Here's how the part is built. I have some questions about the finished solid (model axes, mm). Give positions to 0.01 mm unless a question says otherwise; leave off trailing zeros. Loops run counter-clockwise (first coordinate to the right, second up) from the corner with the lowest first, then second, coordinate; pieces in that order, holes last.
Q1. Suppose I cut it at C-C (x = 75.5). List the corners of the cut face in (y, z) for me (3 decimals).
Q2. I'm going to push flat-ended pins straight in: P1, Ø2, axis at x = 95, y = 1.5, coming from the -Z side; P2, Ø2.5, axis at x = 10.32, z = 0, coming from the +Y side; P3, Ø3, axis at x = -12, y = 0, coming from the +Z side; P4, Ø1, axis at y = 2, z = 62.5, coming from the +X side. Where does each tip first touch, or does it pass through?
Q3. Suppose I cut it at A-A (y = 1.25). Count the separate pieces of the cut face and the enclosed holes in it, and give its area (3 significant figures).
Q4. Thinking about a two-plate mould opening in Y: for faces 1 (the face through (2, -3.175, -2)), 2 (the face through (2, 3.175, -2)), 3 (the face through (-92.73, 0.04, -120.94)), which applies, pulls with the +Y half, pulls with the -Y half, needs draft (parallel to the pull), parting line crosses it, or undercut?
Q5. I need wall thicknesses on probe 1 along X at (y, z) = (-0.25, 0); probe 2 along Z at (x, y) = (87, -1.5); probe 3 along Z at (x, y) = (101.6, 1). Which ranges of each line are inside material? Lowest first, please.
Q6. Suppose I cut it at B-B (z = 65.5). List the corners of the cut face in (x, y) for me (3 decimals).
```python
from build123d import *

# Parameters (mm, degrees)
SKETCH1_R           = 152.4
BOSS_EXTRUDE1_DEPTH = 3.175
SKETCH3_R           = 2.20345
CUT_EXTRUDE1_DEPTH  = 216.619670949
SKETCH5_R           = 1.524
CUT_EXTRUDE3_DEPTH  = 216.619670949


with BuildPart() as part:
    # Sketch1 → Boss-Extrude1 (new, symmetric)
    with BuildSketch(Plane(origin=(0, 0, 0), x_dir=(1, 0, 0), z_dir=(0, 1, 0))):
        with Locations(Location((0, 0, 0), (0, 0, 270))):
            Circle(SKETCH1_R)
    extrude(amount=BOSS_EXTRUDE1_DEPTH, both=True)

    # Sketch3 → Cut-Extrude1 (cut, through all)
    with BuildSketch(Plane(origin=(0, 3.175, 0), x_dir=(1, 0, 0), z_dir=(0, 1, 0))):
        with Locations(Location((-10.31875, 0, 0), (0, 0, 270))):
            Circle(SKETCH3_R)
        with Locations(Location((10.31875, 0, 0), (0, 0, 270))):
            Circle(SKETCH3_R)
        with Locations(Location((66.013427029, 76.332177029, 0), (0, 0, 270))):
            Circle(SKETCH3_R)
        with Locations(Location((86.650927029, 76.332177029, 0), (0, 0, 270))):
            Circle(SKETCH3_R)
        with Locations(Location((-86.650927029, 76.332177029, 0), (0, 0, 270))):
            Circle(SKETCH3_R)
        with Locations(Location((-66.013427029, 76.332177029, 0), (0, 0, 270))):
            Circle(SKETCH3_R)
    extrude(amount=-CUT_EXTRUDE1_DEPTH, mode=Mode.SUBTRACT)

    # Sketch5 → Cut-Extrude3 (cut, through all)
    with BuildSketch(Plane(origin=(0, 3.175, 0), x_dir=(1, 0, 0), z_dir=(0, 1, 0))):
        with Locations(Location((-101.6, 0, 0), (0, 0, 270))):
            Circle(SKETCH5_R)
        with Locations(Location((0, 101.6, 0), (0, 0, 270))):
            Circle(SKETCH5_R)
        with Locations(Location((101.6, 0, 0), (0, 0, 270))):
            Circle(SKETCH5_R)
        with Locations(Location((0, -101.6, 0), (0, 0, 270))):
            Circle(SKETCH5_R)
    extrude(amount=-CUT_EXTRUDE3_DEPTH, mode=Mode.SUBTRACT)


solid = part.part
```
Solutions:
1. outline: (-3.175, -132.384) - (3.175, -132.384) - (3.175, 132.384) - (-3.175, 132.384) - close
2. P1: stops at z = -119.96
2. P2: passes through
2. P3: stops at z = 152.04
2. P4: stops at x = 139.22
3. separate pieces: 1
3. enclosed holes: 10
3. area: 72,800 mm2
4. face 1: pulls with the -Y half
4. face 2: pulls with the +Y half
4. face 3: needs draft
5. probe 1: x = -152.4 to -103.12, -100.08 to -12.52, -8.12 to 8.12, 12.52 to 100.08, 103.12 to 152.4
5. probe 2: z = -125.13 to -78.51, -74.16 to 125.13
5. probe 3: z = -113.59 to -1.52, 1.52 to 113.59
6. outline: (-137.606, -3.175) - (137.606, -3.175) - (137.606, 3.175) - (-137.606, 3.175) - close
